The model under review builds one solid part; all positions refer to its coordinate system, in mm. Face numbers are marked on the shaded views. A direction names the side the tool comes from. Round coordinates to 2 decimals unless told otherwise and drop trailing zeros. Order: outer loops, then holes, each group sorted by start corner. A loop starts at its lowest first (then second) coordinate and runs counter-clockwise, first axis right, second up.
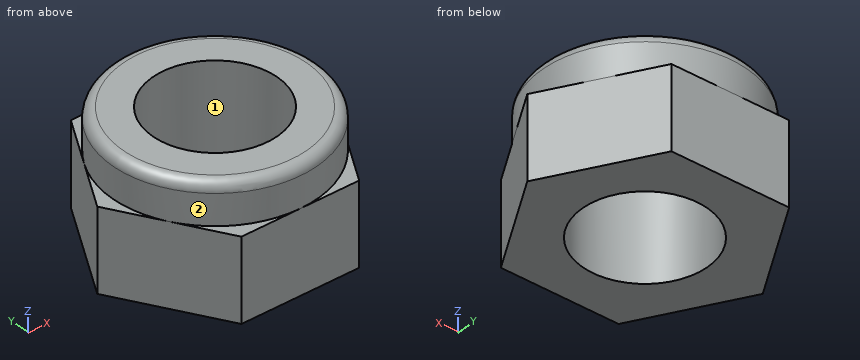
```python
from build123d import *

# Parameters (mm, degrees)
SKETCH1_R           = 3.05
BOSS_EXTRUDE1_DEPTH = 4
SKETCH2_R           = 5
SKETCH2_R_2         = 3.05
BOSS_EXTRUDE2_DEPTH = 2
FILLET1_R           = 0.5


with BuildPart() as part:
    # Sketch1 → Boss-Extrude1 (new body)
    with BuildSketch(Plane.XY):
        Polygon((-2.886751346, -0.1), (-5.773502692, -5.1), (-2.886751346, -10.1), (2.886751346, -10.1), (5.773502692, -5.1), (2.886751346, -0.1), align=None)
        with Locations((0, -5.1)):
            Circle(SKETCH1_R, mode=Mode.SUBTRACT)
    extrude(amount=BOSS_EXTRUDE1_DEPTH)

    # Sketch2 → Boss-Extrude2 (add)
    with BuildSketch(Plane.XY.offset(4)):
        with Locations(Location((0, -5.1, 0), (0, 0, 150))):
            Circle(SKETCH2_R)
        with Locations((0, -5.1)):
            Circle(SKETCH2_R_2, mode=Mode.SUBTRACT)
    extrude(amount=BOSS_EXTRUDE2_DEPTH)

    # Fillet1
    fillet1_edges = [part.edges().sort_by_distance(p)[0] for p in [
        (4.330127019, -7.6, 6),
    ]]
    fillet(fillet1_edges, radius=FILLET1_R)


solid = part.part
```
(1) Consider section A-A (x = 5.25). Write out the cut boundary in (y, z), and give its area (3 significant figures).
Data:
outline: (-6.01, 0) - (-4.19, 0) - (-4.19, 4) - (-6.01, 4) - close
area: 7.25 mm2
(2) To check wall thickness, follow probe 1 along Y at (x, z) = (0, 3.95); probe 2 along X at (y, z) = (-6.25, 4.6); probe 3 along X at (y, z) = (-3.25, 5.45). State the ranges of each line that lie inside material, in increasing order.
Data:
probe 1: y = -10.1 to -8.15, -2.05 to -0.1
probe 2: x = -4.87 to -2.82, 2.82 to 4.87
probe 3: x = -4.65 to -2.42, 2.42 to 4.65
(3) For the marked faces 1 and 2, list the 3-axis set-ups (+Z, -Z, +X, -X, +Y, -Y) from which the entire face can be reached by the end or side of a thin tool; tool diameter is ignored.
Data:
face 1: +Z, -Z
face 2: +Z
(4) Insertion check: pin 1 (2 mm diameter, centred on x = 3, y = -9.5, fed in from +Z); pin 2 (1.5 mm diameter, centred on y = -1, z = 0.5, fed in from +X); pin 3 (5.5 mm diameter, centred on x = 0, y = -5.1, fed in from -Z); pin 4 (1.5 mm diameter, centred on x = 4.5, z = 5, fed in from -Y). Each pin has a flat end and moves straight along its axis. Give the tip position at first contact, or say it passes through.
Data:
pin 1: stops at z = 6
pin 2: stops at x = 3.84
pin 3: passes through
pin 4: stops at y = -8.41
